Read the model definition and answer for the solid it produces. Units are mm, in the model's axes. A direction names the side the tool comes from. Give positions to 0.01 mm unless a question says otherwise; leave off trailing zeros. Order: outer loops, then holes, each group sorted by start corner. A loop starts at its lowest first (then second) coordinate and runs counter-clockwise, first axis right, second up. Notation, with made-up numbers: (-25.75, 40.5) - (22.25, 40.5) arc R15 cw to (22.25, 56.5) - close; hole circle Ø2 at (28, -21.5). An arc over 180 degrees is marked (long way). Use a Markdown table: item, result. Add a question column.
1. A cutting plane is placed at C-C on x = -7. Determine the outline of the cut face in (y, z).
2. Flat-ended cylindrical pins translate along their axes: P1, Ø10.5, axis at x = -37.95, y = -3.96, coming from the +Z side; P2, Ø4.5, axis at x = -37.95, y = -3.96, coming from the +Z side; P3, Ø4, axis at x = -4.5, z = 53, coming from the -Y side; P4, Ø3.5, axis at y = 26.5, z = 56, coming from the -X side. Find the tip coordinate at first contact, or state that the pin passes through.
3. For a pull along X with two mould halves and no side action, classify faces 1 (the flat face through (-39.172, 13.914, 4.93)), 2 (the cylindrical face through (-42.448, -3.762, 9.211)), 3 (the cylindrical face through (8.212, -8.353, 9.211)), 4 (the flat face through (-15, -10.06, 5)) as released by +X, released by -X, zero draft, split by the parting line, or undercut.
4. Which of the six approach directions +Z, -Z, +X, -X, +Y, -Y give full straight-line access (tool end or side, diameter ignored) to faces 5 (the flat face through (-15.382, 27, 46)), 6 (the cylindrical face through (-11.8, 26.6, 57)), 7 (the flat face through (-38, -7, 8.4)), 8 (the flat face through (-4.382, 27, 30))?
5. A cutting plane is placed at A-A on y = -5.5. Determine the outline of the cut face in (x, z), and give its area (3 significant figures).
6. A cutting plane is placed at D-D on y = 25.5. Determine the outline of the cut face in (x, z), and give its area (3 significant figures).
7. Consider L1, parallel to X at y = 23.5, z = 9; L2, parallel to Z at x = -28.5, y = -1; L3, parallel to X at y = 26.5, z = 38.5. Determine where each line is inside the solid, lowest interval first.
8. A cutting plane is placed at B-B on z = 46. Determine the outline of the cut face in (x, y), and give its area (3 significant figures).
```python
from build123d import *

# Parameters (mm, degrees)
BOSS_EXTRUDE1_DEPTH = 10
SKETCH4_R           = 2.75
CUT_EXTRUDE1_DEPTH  = 64.215786076
SKETCH6_R           = 4.5
CUT_EXTRUDE3_DEPTH  = 1.6
SKETCH7_W           = 4
SKETCH7_H           = 8
BOSS_EXTRUDE2_DEPTH = 50
SKETCH8_R           = 3
BOSS_EXTRUDE3_DEPTH = 7
SKETCH9_W           = 5
SKETCH9_H           = 8
CUT_EXTRUDE4_DEPTH  = 82.57703588


with BuildPart() as part:
    # Sketch2 → Boss-Extrude1 (new body)
    with BuildSketch(Plane.XY):
        Polygon((-24.382192178, 22.640051942), (-54.382192178, 4.940051942), (-54.382192178, -10.059948058), (25.617807822, -10.059948058), (25.617807822, 4.940051942), (-4.382192178, 22.640051942), (-4.382192178, 30.640051942), (-24.382192178, 30.640051942), align=None)
    extrude(amount=BOSS_EXTRUDE1_DEPTH)

    # Sketch4 → Cut-Extrude1 (cut, through all)
    with BuildSketch(Plane.XY.offset(10)):
        with Locations((-37.952192178, -3.959948058)):
            Circle(SKETCH4_R)
    cut_extrude1 = extrude(amount=-CUT_EXTRUDE1_DEPTH, mode=Mode.SUBTRACT)

    # Mirror2: Cut-Extrude1 across plane
    add(cut_extrude1.mirror(Plane.ZY.offset(14.382192178)), mode=Mode.SUBTRACT)

    # Sketch6 → Cut-Extrude3 (cut)
    with BuildSketch(Plane.XY.offset(10)):
        with Locations((-37.952192178, -3.959948058)):
            Circle(SKETCH6_R)
        with Locations((9.187807822, -3.959948058)):
            Circle(SKETCH6_R)
    extrude(amount=-CUT_EXTRUDE3_DEPTH, mode=Mode.SUBTRACT)

    # Sketch7 → Boss-Extrude2 (add)
    with BuildSketch(Plane.XY.offset(10)):
        with Locations((-6.382192178, 26.640051942)):
            Rectangle(SKETCH7_W, SKETCH7_H)
    extrude(amount=BOSS_EXTRUDE2_DEPTH)

    # Sketch8 → Boss-Extrude3 (add)
    with BuildSketch(Plane.ZY.offset(8.382192178)):
        with Locations(Location((54, 26.640051942, 0), (0, 0, 180))):
            Circle(SKETCH8_R)
        with Locations(Location((46, 26.640051942, 0), (0, 0, 180))):
            Circle(SKETCH8_R)
    extrude(amount=BOSS_EXTRUDE3_DEPTH)

    # Sketch9 → Cut-Extrude4 (cut, through all)
    with BuildSketch(Plane.ZY.offset(8.382192178)):
        with Locations((50, 26.640051942)):
            Rectangle(SKETCH9_W, SKETCH9_H)
    extrude(amount=CUT_EXTRUDE4_DEPTH, mode=Mode.SUBTRACT)


solid = part.part
```
Output values:
| question | item | result |
|---|---|---|
| 1 | outline | (-10.06, 0) - (30.64, 0) - (30.64, 60) - (22.64, 60) - (22.64, 10) - (-10.06, 10) - close |
| 2 | P1 | z = 10 |
| 2 | P2 | through |
| 2 | P3 | y = 22.64 |
| 2 | P4 | x = -15.38 |
| 3 | face 1 | released by -X |
| 3 | face 2 | undercut |
| 3 | face 3 | undercut |
| 3 | face 4 | zero draft |
| 4 | face 5 | +Z, -X, +Y, -Y |
| 4 | face 6 | -X |
| 4 | face 7 | +Z |
| 4 | face 8 | +Z, -Z, +X, +Y |
| 5 | outline | (-54.38, 0) - (-40.23, 0) - (-40.23, 8.4) - (-42.18, 8.4) - (-42.18, 10) - (-54.38, 10) - close; (-35.67, 0) - (6.91, 0) - (6.91, 8.4) - (4.96, 8.4) - (4.96, 10) - (-33.72, 10) - (-33.72, 8.4) - (-35.67, 8.4) - close; (11.47, 0) - (25.62, 0) - (25.62, 10) - (13.42, 10) - (13.42, 8.4) - (11.47, 8.4) - close |
| 5 | area | 696 mm² |
| 6 | outline | (-24.38, 0) - (-4.38, 0) - (-4.38, 60) - (-8.38, 60) - (-8.38, 56.77) - (-15.38, 56.77) - (-15.38, 52.5) - (-8.38, 52.5) - (-8.38, 47.5) - (-15.38, 47.5) - (-15.38, 43.23) - (-8.38, 43.23) - (-8.38, 10) - (-24.38, 10) - close |
| 6 | area | 460 mm² |
| 7 | L1 | -24.38 to -4.38 |
| 7 | L2 | 0 to 10 |
| 7 | L3 | -8.38 to -4.38 |
| 8 | outline | (-15.38, 23.64) - (-8.38, 23.64) - (-8.38, 22.64) - (-4.38, 22.64) - (-4.38, 30.64) - (-8.38, 30.64) - (-8.38, 29.64) - (-15.38, 29.64) - close |
| 8 | area | 74.0 mm² |
